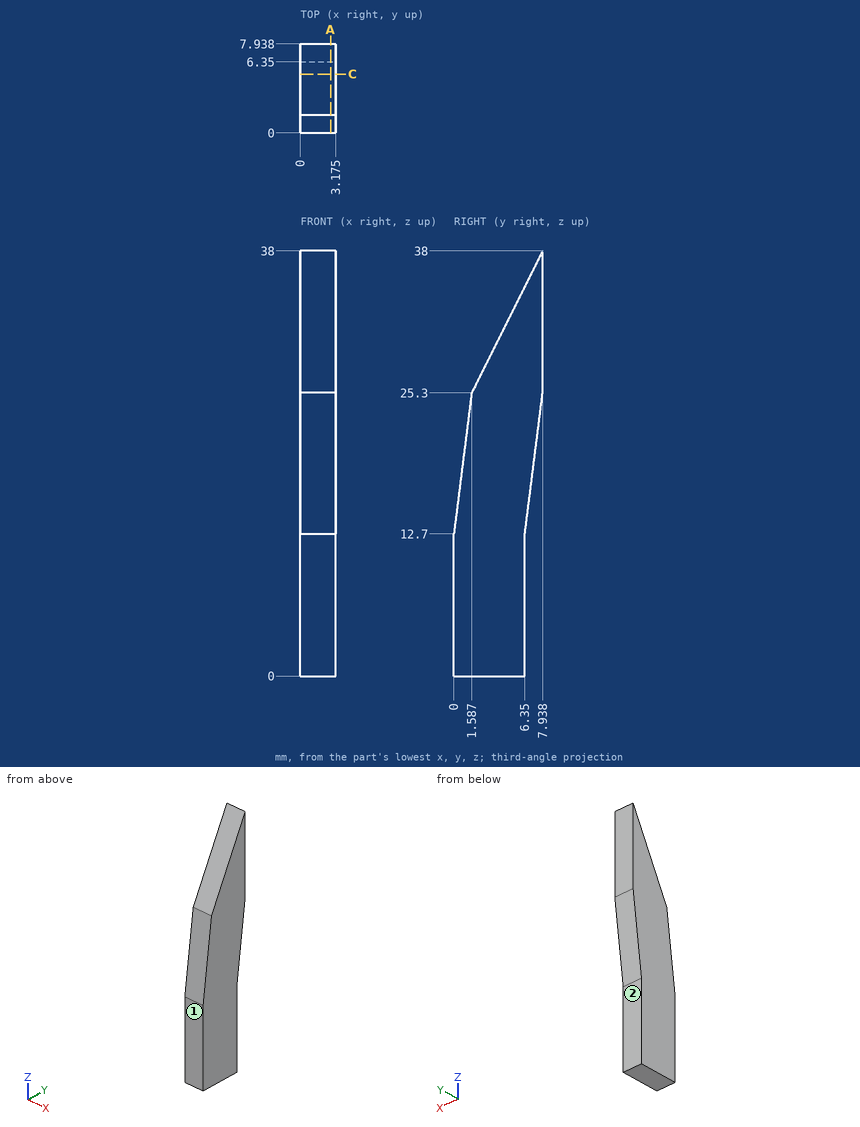
Could you check a few things on this drawing? It's one solid part, dimensions in mm from its lowest x, y, z. A direction names the side the tool comes from. Coordinates: 2 decimals unless noted, no trailing zeros. Loops run counter-clockwise (first coordinate to the right, second up) from the corner with the lowest first, then second, coordinate; pieces in that order, holes last. Notation, with made-up numbers: (56, -6.5) - (80, -6.5) arc R14 ccw to (80, -2.5) - close; hole circle Ø5 at (80.25, 78). An arc over 180 degrees is marked (long way). Return JSON: item names as keys, results as strings. Group by question number.
Item 1: I need wall thicknesses on line 1 (Y direction, x = 1.2, z = 6.5); line 2 (Z direction, x = 1.85, y = 4.75) (1 decimal); line 3 (Z direction, x = 2.3, y = 5.5) (1 decimal). Which ranges of each line are inside material? Lowest first, please. Write a range as from..to.
Item 2: Will these pins go through, and if not, where does the flat tip stop? P1, Ø1.5, axis at x = 2.5, y = 6, coming from the +Z side (1 decimal); P2, Ø1.6, axis at x = 2, z = 4.5, coming from the +Y side.
Item 3: If we section it at A-A on x = 2.7: Write out the boundary of the cut face in (y, z), and give its area (3 significant figures).
Item 4: On a 3-axis mill with a long thin cutter (end or side, diameter ignored), from which of +Z, -Z, +X, -X, +Y, -Y can I reach the whole of each face in a straight line? I mean the marked faces 1 and 2. Say none if no direction works.
Item 5: If we section it at C-C on y = 5.25: Write out the boundary of the cut face in (x, z) (1 decimal).
Calculated:
{
 "1": {"line 1": "y = 0..6.35", "line 2": "z = 0..31.6", "line 3": "z = 0..33.1"},
 "2": {"P1": "stops at z = 35.6", "P2": "stops at y = 6.35"},
 "3": {"outline": "(0, 0) - (6.35, 0) - (6.35, 12.7) - (7.94, 25.3) - (7.94, 38) - (1.59, 25.3) - (0, 12.7) - close", "area": "201 mm^2"},
 "4": {"face 1": "+Z, -Z, +X, -X, -Y", "face 2": "-Z, +X, -X, +Y"},
 "5": {"outline": "(0, 0) - (3.2, 0) - (3.2, 32.6) - (0, 32.6) - close"}
}
